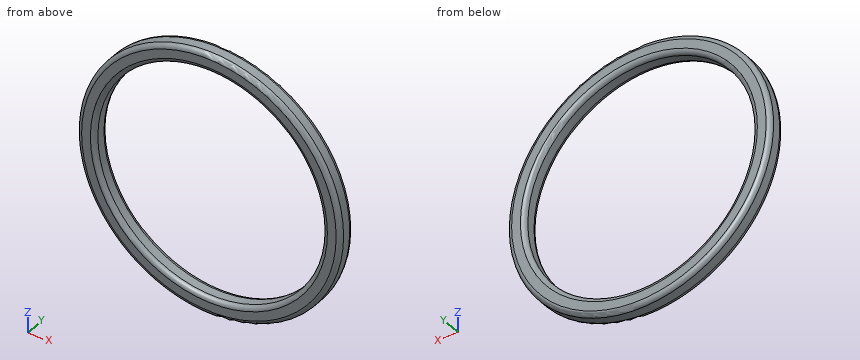
```python
from build123d import *

# Parameters (mm, degrees)
F0_R     = 19.05
F0_R_2   = 16.51
F1_DEPTH = 2.54
F2_R     = 0.635
F3_R     = 0.635


with BuildPart() as f1:
    # F0 (on Front) → F1 (new body)
    with BuildSketch(Plane.XZ):
        Circle(F0_R)
        Circle(F0_R_2, mode=Mode.SUBTRACT)
    extrude(amount=F1_DEPTH)

    # F2
    f2_edges = [f1.edges().sort_by_distance(p)[0] for p in [
        (-16.51, 0, 0),
        (-19.05, 0, 0),
    ]]
    fillet(f2_edges, radius=F2_R)

    # F3
    f3_edges = [f1.edges().sort_by_distance(p)[0] for p in [
        (-16.51, -2.54, 0),
        (-19.05, -2.54, 0),
    ]]
    fillet(f3_edges, radius=F3_R)


solid = f1.part
```
Verification items for the finished model (mm, model axes). Round coordinates to 2 decimals unless told otherwise and drop trailing zeros. Write each loop counter-clockwise with the first axis right and the second up, starting at its lowest first coordinate (ties: lowest second). Pieces come first, ordered by that corner, then holes.
1. Gauge pin test, flat ends, axial feed: P1, Ø1.5, axis at y = -1, z = -9.5, coming from the +X side; P2, Ø1, axis at x = 12, z = -10.5, coming from the -Y side; P3, Ø1, axis at x = -2, y = -1.5, coming from the +Z side. Record the tip position at first contact, or that the pin passes through.
2. Scan lines: L1, parallel to Z at x = 0, y = -1.25; L2, parallel to X at y = -0.15, z = 3.5; L3, parallel to Z at x = 1.5, y = -1.85. Record each from-to range of solid material in increasing order.
3. Section check B-B on x = 0. Enter the section's corners in (y, z) (3 decimals), plus the area to 3 significant figures.
4. Section check C-C on y = -1.4. Enter the section's corners in (x, z), plus the area to 3 significant figures.
5. Section check A-A on z = 0. Enter the section's corners in (x, y) (3 decimals).
Answer:
1. P1: stops at x = 16.92
1. P2: passes through
1. P3: stops at z = 18.99
2. L1: z = -19.05 to -16.51, 16.51 to 19.05
2. L2: x = -18.5 to -16.37, 16.37 to 18.5
2. L3: z = -18.99 to -16.44, 16.44 to 18.99
3. outline: (-2.54, -18.415) arc R0.635 ccw to (-1.905, -19.05) - (-0.635, -19.05) arc R0.635 ccw to (0, -18.415) - (0, -17.145) arc R0.635 ccw to (-0.635, -16.51) - (-1.905, -16.51) arc R0.635 ccw to (-2.54, -17.145) - close; (-2.54, 17.145) arc R0.635 ccw to (-1.905, 16.51) - (-0.635, 16.51) arc R0.635 ccw to (0, 17.145) - (0, 18.415) arc R0.635 ccw to (-0.635, 19.05) - (-1.905, 19.05) arc R0.635 ccw to (-2.54, 18.415) - close
3. area: 12.2 mm2
4. outline: circle Ø38.1 at (0, 0); hole circle Ø33.02 at (0, 0)
4. area: 284 mm2
5. outline: (-19.05, -1.905) arc R0.635 ccw to (-18.415, -2.54) - (-17.145, -2.54) arc R0.635 ccw to (-16.51, -1.905) - (-16.51, -0.635) arc R0.635 ccw to (-17.145, 0) - (-18.415, 0) arc R0.635 ccw to (-19.05, -0.635) - close; (16.51, -1.905) arc R0.635 ccw to (17.145, -2.54) - (18.415, -2.54) arc R0.635 ccw to (19.05, -1.905) - (19.05, -0.635) arc R0.635 ccw to (18.415, 0) - (17.145, 0) arc R0.635 ccw to (16.51, -0.635) - close
